Study the drawing (mm; zero at the part's minimum x, y, z) and answer. Coordinates: 2 decimals unless noted, no trailing zeros. Order: outer loops, then holes, each group sorted by start corner. A loop starts at its lowest first (then second) coordinate and runs counter-clockwise, first axis right, second up. Notation, with made-up numbers: (39, 40.5) -> (43, 40.5) arc R11 cw to (43, 57.5) -> close; hole circle Ø3 at (-15.5, -33.5). An arc over 180 degrees is marked (long way). Answer as CSV lines item,"result". Start each with the question number.
Item 1: Each of these flat-tipped pins is pushed along its axis until it touches: pin 1 Ø5.5 at (x, z) = (7.5, 4) entering from -Y; pin 2 Ø0.8 at (x, y) = (14.5, 6.5) entering from +Z; pin 3 Ø0.8 at (x, y) = (14.5, 10) entering from -Z; pin 4 Ø2 at (x, y) = (4.5, 3.5) entering from +Z. Where does it stop, or does it pass through?
Item 2: Straight lines are drawn through the part: L1, parallel to Z at x = 7.5, y = 14.8; L2, parallel to Y at x = 9, z = 10; L3, parallel to X at y = 1.9, z = 4. For each, find the intervals that lie inside material, in ascending order.
Item 3: Section A-A (y = 3.75) is taken. Write down the section's boundary in (x, z), then the cut area to 3 significant figures.
Item 4: For a pull along X with two mould halves and no side action, classify the marked faces 1, 2 and 3 as pulls with the +X half, pulls with the -X half, needs draft (parallel to the pull), parting line crosses it, or undercut.
Item 5: Section C-C (z = 31.5) is taken. Write down the section's boundary in (x, y).
Item 6: Section D-D (y = 13.5) is taken. Write down the section's boundary in (x, z), then the cut area to 3 significant figures.
Item 7: Section B-B (x = 7.5) is taken. Write down the section's boundary in (y, z).
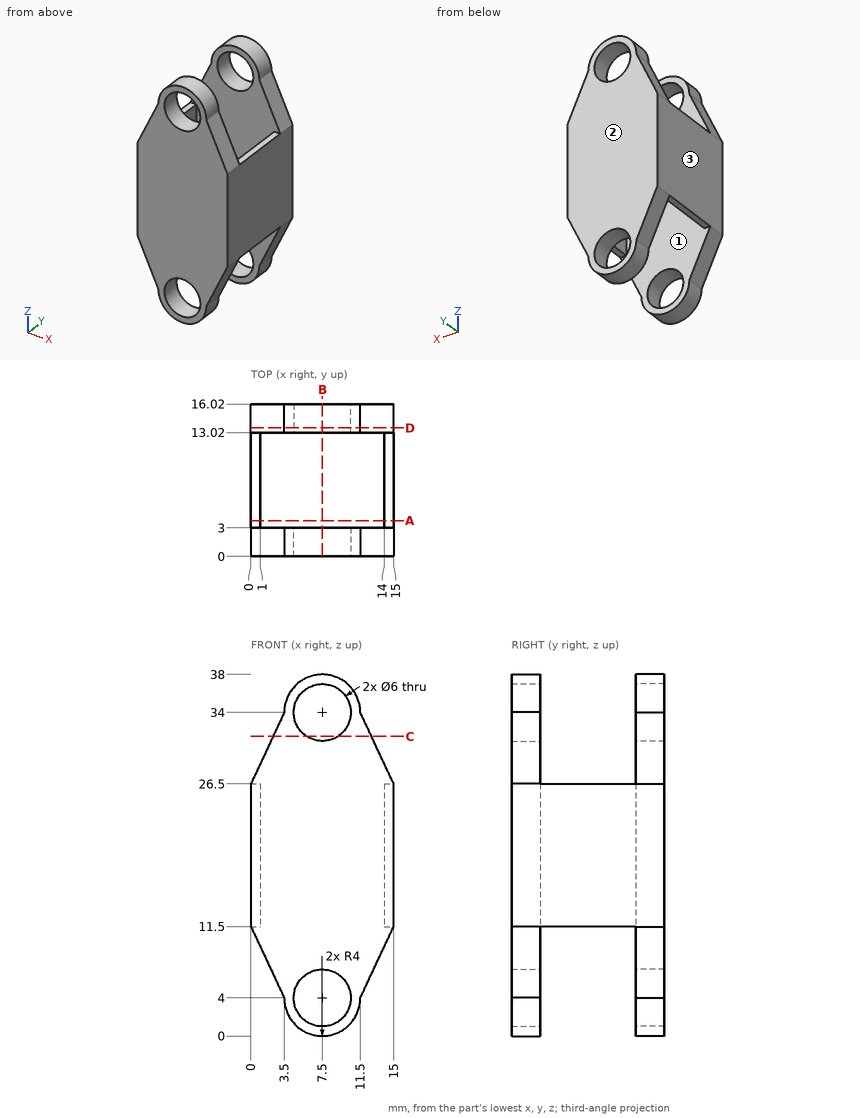
Checked values:
1,pin 1,"passes through"
1,pin 2,"stops at z = 26.5"
1,pin 3,"stops at z = 11.5"
1,pin 4,"stops at z = 37.38"
2,L1,"z = 0 to 1, 7 to 31, 37 to 38"
2,L2,"y = 0 to 3, 13.02 to 16.02"
2,L3,"x = 3.5 to 4.5, 10.5 to 11.5"
3,outline,"(0, 11.5) -> (1, 11.5) -> (1, 26.5) -> (0, 26.5) -> close; (14, 11.5) -> (15, 11.5) -> (15, 26.5) -> (14, 26.5) -> close"
3,area,"30.0 mm^2"
4,face 1,"undercut"
4,face 2,"needs draft"
4,face 3,"pulls with the -X half"
5,outline,"(2.33, 0) -> (5.84, 0) -> (5.84, 3) -> (2.33, 3) -> close; (2.33, 13.02) -> (5.84, 13.02) -> (5.84, 16.02) -> (2.33, 16.02) -> close; (9.16, 0) -> (12.67, 0) -> (12.67, 3) -> (9.16, 3) -> close; (9.16, 13.02) -> (12.67, 13.02) -> (12.67, 16.02) -> (9.16, 16.02) -> close"
6,outline,"(0, 11.5) -> (3.5, 4) arc R4 ccw to (11.5, 4) -> (15, 11.5) -> (15, 26.5) -> (11.5, 34) arc R4 ccw to (3.5, 34) -> (0, 26.5) -> close; hole circle Ø6 at (7.5, 4); hole circle Ø6 at (7.5, 34)"
6,area,"391 mm^2"
7,outline,"(0, 0) -> (3, 0) -> (3, 1) -> (0, 1) -> close; (0, 7) -> (3, 7) -> (3, 31) -> (0, 31) -> close; (0, 37) -> (3, 37) -> (3, 38) -> (0, 38) -> close; (13.02, 0) -> (16.02, 0) -> (16.02, 1) -> (13.02, 1) -> close; (13.02, 7) -> (16.02, 7) -> (16.02, 31) -> (13.02, 31) -> close; (13.02, 37) -> (16.02, 37) -> (16.02, 38) -> (13.02, 38) -> close"
